from build123d import *

# Parameters (mm, degrees)
SKETCH_1_R          = 27.5
SKETCH_1_R_2        = 19.5
EXTRUDE_1_DEPTH     = 92
EXTRUDE_START       = -15
SKETCH_2_R          = 10
EXTRUDE_2_DEPTH     = 15
CUT_EXTRUDE_1_REACH = 153.118
SKETCH_3_W          = 5
SKETCH_3_H          = 48
EXTRUDE_START_2     = 56
EXTRUDE_3_DEPTH     = 56
FILLET_1_R          = 10
CUT_EXTRUDE_2_REACH = 153.118
SKETCH_7_R          = 4


with BuildPart() as part:
    # 草图1 → 凸台-拉伸1 (new body)
    with BuildSketch(Plane(origin=(0, 0, 0), x_dir=(0, 0, -1), z_dir=(1, 0, 0))):
        Circle(SKETCH_1_R)
        Circle(SKETCH_1_R_2, mode=Mode.SUBTRACT)
    extrude(amount=EXTRUDE_1_DEPTH)

    # 草图2 → 凸台-拉伸2 (add)
    with BuildSketch(Plane(origin=(92, 0, 0), x_dir=(0, 0, -1), z_dir=(1, 0, 0)).offset(EXTRUDE_START)):
        with BuildLine():
            Line((-19, 19.880895352), (-19, 91.5))
            ThreePointArc((-19, 91.5), (0, 110.5), (19, 91.5))
            Line((19, 91.5), (19, 19.880895352))
            ThreePointArc((19, 19.880895352), (0, 27.5), (-19, 19.880895352))
        make_face()
        with Locations((0, 91.5)):
            Circle(SKETCH_2_R, mode=Mode.SUBTRACT)
    extrude(amount=EXTRUDE_2_DEPTH)

    # 草图3 → 切除-拉伸1 (cut, up to next)
    with BuildSketch(Plane.XY.offset(19), mode=Mode.PRIVATE) as cut_extrude_1_sk1:
        with Locations((79.5, 86.5)):
            Rectangle(SKETCH_3_W, SKETCH_3_H)
    cut_extrude_1_tool1 = extrude(cut_extrude_1_sk1.sketch, amount=-CUT_EXTRUDE_1_REACH, mode=Mode.PRIVATE) & part.part
    add(cut_extrude_1_tool1.solids().sort_by_distance((79.5, 86.5, 19))[0], mode=Mode.SUBTRACT)

    # 草图6 → 凸台-拉伸3 (add)
    with BuildSketch(Plane.ZY.offset(-77).offset(EXTRUDE_START_2)):
        with BuildLine():
            Line((19, 19.880895352), (19, 52.5))
            Line((19, 52.5), (9, 52.5))
            Line((9, 52.5), (9, 25.98557292))
            ThreePointArc((9, 25.98557292), (14.328878953, 23.471966853), (19, 19.880895352))
        make_face()
    extrude(amount=-EXTRUDE_3_DEPTH)

    # 圆角1
    fillet_1_edges = [part.edges().sort_by_distance(p)[0] for p in [
        (21, 52.5, 14),
    ]]
    fillet(fillet_1_edges, radius=FILLET_1_R)

    # 草图7 → 切除-拉伸2 (cut, up to next)
    with BuildSketch(Plane.XY.offset(19), mode=Mode.PRIVATE) as cut_extrude_2_sk1:
        with Locations((31, 42.5)):
            Circle(SKETCH_7_R)
    cut_extrude_2_tool1 = extrude(cut_extrude_2_sk1.sketch, amount=-CUT_EXTRUDE_2_REACH, mode=Mode.PRIVATE) & part.part
    add(cut_extrude_2_tool1.solids().sort_by_distance((31, 42.5, 19))[0], mode=Mode.SUBTRACT)


solid = part.part
Verification items for the finished model (mm, model axes). A direction names the side the tool comes from. Round coordinates to 2 decimals unless told otherwise and drop trailing zeros. Loops run counter-clockwise (first coordinate to the right, second up) from the corner with the lowest first, then second, coordinate; pieces in that order, holes last. Notation, with made-up numbers: (-29, 87.5) - (16, 87.5) arc R19 ccw to (16, 92.5) - close; hole circle Ø8 at (37, 24). An arc over 180 degrees is marked (long way). Answer in a Markdown table with one row per item. Add a question column.
Q1. Tool access check on faces 5 (the face through (86, 56, -19)), 6 (the face through (21, 34, 14)), 7 (the face through (0, 19, -6)), 8 (the face through (79, 62.5, 0)), 9 (the face through (45.356, -26.846, 5.961)). Record the directions out of +Z, -Z, +X, -X, +Y, -Y that give a thin tool (end or side, any length) a straight path to the whole face; none if there is none.
Q2. Release check for a two-part mould opening along Z. For faces 1 (the face through (45.356, 19.334, 2.539)), 2 (the face through (82, 81, 0)), 3 (the face through (86.93, 101.415, 1.302)), 4 (the face through (64, 39, 19)) record: pulls with the +Z half, pulls with the -Z half, needs draft (parallel to the pull), parting line crosses it, or undercut.
Q3. Gauge pin test, flat ends, axial feed: pin 1 (8 mm diameter, centred on x = 48, y = 37.5, fed in from -Z); pin 2 (6 mm diameter, centred on x = 24.5, z = 15, fed in from +Y); pin 3 (16.5 mm diameter, centred on x = 87, y = 67, fed in from -Z); pin 4 (5 mm diameter, centred on x = 31, y = 42.5, fed in from -Z). Record the tip position at first contact, or that the pin passes through.
Q4. Material ranges on line 1 (Y direction, x = 84, z = 0); line 2 (Y direction, x = 31, z = 12); line 3 (Y direction, x = 54, z = 0), recorded low to high.
Q5. Section check A-A on y = 0. Enter the section's corners in (x, z).
Q6. Section check D-D on z = 14. Enter the section's corners in (x, y), plus the area to 3 significant figures.
Q7. Section check C-C on x = 80.5. Enter the section's corners in (y, z), plus the area to 3 significant figures.
Q8. Section check B-B on z = 0. Enter the section's corners in (x, y).
Found:
| question | item | result |
|---|---|---|
| 1 | face 5 | -Z, +X, -X, +Y |
| 1 | face 6 | +Z, -X, +Y |
| 1 | face 7 | +Z, -Z, -X, +Y, -Y |
| 1 | face 8 | +Z, -Z, -X, +Y |
| 1 | face 9 | -X |
| 2 | face 1 | undercut |
| 2 | face 2 | needs draft |
| 2 | face 3 | undercut |
| 2 | face 4 | pulls with the +Z half |
| 3 | pin 1 | stops at z = 9 |
| 3 | pin 2 | stops at y = 51.87 |
| 3 | pin 3 | stops at z = -19 |
| 3 | pin 4 | passes through |
| 4 | line 1 | y = -27.5 to -19.5, 19.5 to 81.5, 101.5 to 110.5 |
| 4 | line 2 | y = -24.74 to -15.37, 15.37 to 38.5, 46.5 to 52.5 |
| 4 | line 3 | y = -27.5 to -19.5, 19.5 to 27.5 |
| 5 | outline | (0, -27.5) - (92, -27.5) - (92, -19.5) - (0, -19.5) - close; (0, 19.5) - (92, 19.5) - (92, 27.5) - (0, 27.5) - close |
| 6 | outline | (0, -23.67) - (92, -23.67) - (92, -13.57) - (0, -13.57) - close; (0, 13.57) - (92, 13.57) - (92, 104.35) - (82, 104.35) - (82, 62.5) - (77, 62.5) - (77, 52.5) - (31, 52.5) arc R10 ccw to (21, 42.5) - (21, 23.67) - (0, 23.67) - close; hole circle Ø8 at (31, 42.5) |
| 6 | area | 4,400 mm² |
| 7 | outline | (19.88, -19) - (62.5, -19) - (62.5, 19) - (19.88, 19) arc R27.5 ccw (long way) to start; hole circle Ø39 at (0, 0) |
| 7 | area | 2,600 mm² |
| 8 | outline | (0, -27.5) - (92, -27.5) - (92, -19.5) - (0, -19.5) - close; (0, 19.5) - (92, 19.5) - (92, 81.5) - (82, 81.5) - (82, 62.5) - (77, 62.5) - (77, 27.5) - (0, 27.5) - close; (82, 101.5) - (92, 101.5) - (92, 110.5) - (82, 110.5) - close |
